Source: CAD feature listing. Evaluate the final solid. Frame: model axes, mm. Face numbers are marked on the shaded views. A direction names the side the tool comes from. Give positions to 0.01 mm unless a question says otherwise; leave off trailing zeros. Loops run counter-clockwise (first coordinate to the right, second up) from the corner with the lowest first, then second, coordinate; pieces in that order, holes last. Notation, with made-up numbers: (-17.75, 29) -> (30.25, 29) arc R16 cw to (30.25, 47) -> close; hole circle Ø8 at (51, 17). An arc over 180 degrees is marked (long way). Return JSON: item names as keys, results as strings. Group by question number.
(1) Cut plane C-C on z = 12.5. Return loops of the section in (x, y).
(2) Cut plane B-B on x = 18. Return loops of the section in (y, z).
(3) Ray query, line 1 (Z direction, x = 26.5, y = 9.5); line 2 (X direction, y = 4.75, z = 27); line 3 (X direction, y = 7.5, z = 51). Return the intervals inside material, ascending. Write a range as from..to.
(4) Cut plane A-A on z = 24.5. Return loops of the section in (x, y), then the cut area to 3 significant figures.
(5) Access query for the marked faces 1, 2, 3, 4 and 5. Directions: +Z, -Z, +X, -X, +Y, -Y. A direction counts if a zero-diameter tool reaches every point of the face in a straight line with its end or side. Return the directions, or none.
(6) Pin query (flat end, axial travel): pin 1 (5 mm diameter, centred on y = 2.5, z = 52.5, fed in from -X); pin 2 (2 mm diameter, centred on x = 33, y = 4, fed in from +Z); pin 3 (1.6 mm diameter, centred on x = 14, z = 55.5, fed in from +Y). Return the tip coordinate at first contact, or that it passes through.
(7) Cut plane D-D on x = -8. Return loops of the section in (y, z).
(8) Draft query along Z for the marked faces 6, 7 and 8. Return one class per face: released by +Z, released by -Z, zero draft, split by the parting line, or undercut.
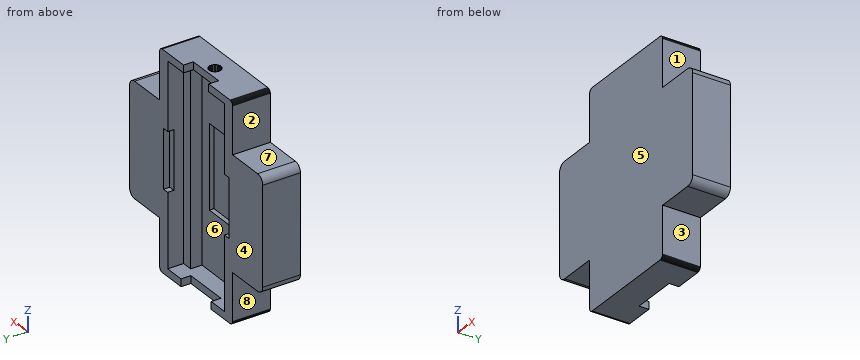
```python
from build123d import *

# Parameters (mm, degrees)
BOSS_EXTRUDE1_DEPTH = 9.999999776
SKETCH2_W           = 17.000000924
SKETCH2_H           = 52.999999374
CUT_EXTRUDE1_DEPTH  = 7.199999876
CUT_EXTRUDE2_REACH  = 66.216
SKETCH4_W           = 2.799998969
SKETCH4_H           = 52.999999374
CUT_EXTRUDE3_REACH  = 66.216
SKETCH6_W           = 2.7999999
SKETCH6_H           = 52.999999374
CUT_EXTRUDE4_REACH  = 66.73
SKETCH7_W           = 10.000000707
SKETCH7_H           = 2.599999774
CUT_EXTRUDE5_REACH  = 66.73
SKETCH8_W           = 12.000000104
SKETCH8_H           = 2.599999774
CUT_EXTRUDE6_DEPTH  = 63.976185295
SKETCH10_W          = 1.699999906
SKETCH10_H          = 15.499999747
CUT_EXTRUDE7_DEPTH  = 1.600000076
SKETCH11_W          = 1.700000837
SKETCH11_H          = 15.499999747
CUT_EXTRUDE8_DEPTH  = 1.600000076
SKETCH12_W          = 11.099998839
SKETCH12_H          = 22.099997848
CUT_EXTRUDE9_DEPTH  = 1.199999941
SKETCH13_W          = 30
SKETCH13_H          = 9.999999776
BOSS_EXTRUDE2_DEPTH = 12
SKETCH14_W          = 30
SKETCH14_H          = 9.999999776
BOSS_EXTRUDE3_DEPTH = 12
FILLET1_R           = 2


with BuildPart() as part:
    # Sketch1 → Boss-Extrude1 (new body)
    with BuildSketch(Plane.XZ):
        Polygon((0.84356498, 0.012312084), (0.999999233, 0), (28.000000864, 0), (28.156435117, 0.012312084), (28.30901742, 0.048942864), (28.453988954, 0.108992681), (28.587784618, 0.190982595), (28.707107529, 0.292893499), (28.80901657, 0.412214547), (28.891006485, 0.546010211), (28.951056302, 0.690983608), (28.987688944, 0.843565969), (28.999999166, 1.000000164), (28.999999166, 56.000001729), (28.987688944, 56.156434119), (28.951056302, 56.309018284), (28.891006485, 56.453991681), (28.80901657, 56.587785482), (28.707107529, 56.707106531), (28.587784618, 56.809015572), (28.453988954, 56.891005486), (28.30901742, 56.951057166), (28.156435117, 56.987687945), (28.000000864, 57.00000003), (0.999999233, 57.00000003), (0.84356498, 56.987687945), (0.690982677, 56.951057166), (0.54600928, 56.891005486), (0.412214547, 56.809015572), (0.292892568, 56.707106531), (0.190982595, 56.587785482), (0.108992681, 56.453991681), (0.048942864, 56.309018284), (0.012311153, 56.156434119), (0, 56.000001729), (0, 1.000000164), (0.012311153, 0.843565969), (0.048942864, 0.690983608), (0.108992681, 0.546010211), (0.190982595, 0.412214547), (0.292892568, 0.292893499), (0.412214547, 0.190982595), (0.54600928, 0.108992681), (0.690982677, 0.048942864), align=None)
    extrude(amount=-BOSS_EXTRUDE1_DEPTH)

    # Sketch2 → Cut-Extrude1 (cut)
    with BuildSketch(Plane(origin=(0, 9.999999776, 0), x_dir=(-1, 0, 0), z_dir=(0, 1, 0))):
        with Locations((-14.499999583, 28.500000015)):
            Rectangle(SKETCH2_W, SKETCH2_H)
    extrude(amount=-CUT_EXTRUDE1_DEPTH, mode=Mode.SUBTRACT)

    # Sketch4 → Cut-Extrude2 (cut, up to next)
    with BuildSketch(Plane.XZ.offset(-5.799999926), mode=Mode.PRIVATE) as cut_extrude2_sk1:
        with Locations((24.39999953, 28.500000015)):
            Rectangle(SKETCH4_W, SKETCH4_H)
    cut_extrude2_tool1 = extrude(cut_extrude2_sk1.sketch, amount=-CUT_EXTRUDE2_REACH, mode=Mode.PRIVATE) & part.part
    add(cut_extrude2_tool1.solids().sort_by_distance((24.4, 5.8, 28.5))[0], mode=Mode.SUBTRACT)

    # Sketch6 → Cut-Extrude3 (cut, up to next)
    with BuildSketch(Plane.XZ.offset(-5.799999926), mode=Mode.PRIVATE) as cut_extrude3_sk1:
        with Locations((4.599999171, 28.500000015)):
            Rectangle(SKETCH6_W, SKETCH6_H)
    cut_extrude3_tool1 = extrude(cut_extrude3_sk1.sketch, amount=-CUT_EXTRUDE3_REACH, mode=Mode.PRIVATE) & part.part
    add(cut_extrude3_tool1.solids().sort_by_distance((4.599999, 5.8, 28.5))[0], mode=Mode.SUBTRACT)

    # Sketch7 → Cut-Extrude4 (cut, up to next)
    with BuildSketch(Plane.XY.offset(57.00000003), mode=Mode.PRIVATE) as cut_extrude4_sk1:
        with Locations((14.500000049, 8.699999889)):
            Rectangle(SKETCH7_W, SKETCH7_H)
    cut_extrude4_tool1 = extrude(cut_extrude4_sk1.sketch, amount=-CUT_EXTRUDE4_REACH, mode=Mode.PRIVATE) & part.part
    add(cut_extrude4_tool1.solids().sort_by_distance((14.5, 8.7, 57))[0], mode=Mode.SUBTRACT)

    # Sketch8 → Cut-Extrude5 (cut, up to next)
    with BuildSketch(Plane(origin=(0, 0, 0), x_dir=(-1, 0, 0), z_dir=(0, 0, -1)), mode=Mode.PRIVATE) as cut_extrude5_sk1:
        with Locations((-14.500000514, 8.699999889)):
            Rectangle(SKETCH8_W, SKETCH8_H)
    cut_extrude5_tool1 = extrude(cut_extrude5_sk1.sketch, amount=-CUT_EXTRUDE5_REACH, mode=Mode.PRIVATE) & part.part
    add(cut_extrude5_tool1.solids().sort_by_distance((14.500001, 8.7, 0))[0], mode=Mode.SUBTRACT)

    # Sketch9 → Cut-Extrude6 (cut, through all)
    with BuildSketch(Plane(origin=(0, 0, 54.999999702), x_dir=(-1, 0, 0), z_dir=(0, 0, -1))):
        Polygon((-16.008604318, 4.466976505), (-15.896821395, 4.219688009), (-15.74485749, 3.994848114), (-15.557079576, 3.798924387), (-15.338891186, 3.637553426), (-15.096570365, 3.515377408), (-14.837087132, 3.435911611), (-14.567905106, 3.401441732), (-14.296771027, 3.412959399), (-14.03148286, 3.470133292), (-13.779673725, 3.571318695), (-13.548586518, 3.713604528), (-13.344869949, 3.892897861), (-13.174383901, 4.104040563), (-13.042034581, 4.34095785), (-12.951626442, 4.596835002), (-12.905763462, 4.86431038), (-12.905763462, 5.135689396), (-12.951626442, 5.403164774), (-13.042034581, 5.659041926), (-13.174383901, 5.895959679), (-13.344869949, 6.107102148), (-13.548586518, 6.286395248), (-13.779673725, 6.428681314), (-14.03148286, 6.529866718), (-14.296771027, 6.587040611), (-14.567905106, 6.598558277), (-14.837087132, 6.564088166), (-15.096570365, 6.484622601), (-15.338891186, 6.362446584), (-15.557079576, 6.201075856), (-15.74485749, 6.005152129), (-15.896821395, 5.780311767), (-16.008604318, 5.533023737), (-16.076983884, 5.270401482), (-16.10000059, 4.999999888), (-16.076983884, 4.729599226), align=None)
    extrude(amount=-CUT_EXTRUDE6_DEPTH, mode=Mode.SUBTRACT)

    # Sketch10 → Cut-Extrude7 (cut)
    with BuildSketch(Plane(origin=(0, 9.999999776, 0), x_dir=(-1, 0, 0), z_dir=(0, 1, 0))):
        with Locations((-2.349999268, 29.250000603)):
            Rectangle(SKETCH10_W, SKETCH10_H)
    extrude(amount=-CUT_EXTRUDE7_DEPTH, mode=Mode.SUBTRACT)

    # Sketch11 → Cut-Extrude8 (cut)
    with BuildSketch(Plane(origin=(0, 9.999999776, 0), x_dir=(-1, 0, 0), z_dir=(0, 1, 0))):
        with Locations((-26.649999433, 29.250000603)):
            Rectangle(SKETCH11_W, SKETCH11_H)
    extrude(amount=-CUT_EXTRUDE8_DEPTH, mode=Mode.SUBTRACT)

    # Sketch12 → Cut-Extrude9 (cut)
    with BuildSketch(Plane(origin=(0, 2.7999999, 0), x_dir=(-1, 0, 0), z_dir=(0, 1, 0))):
        with Locations((-14.499999117, 28.500000015)):
            Rectangle(SKETCH12_W, SKETCH12_H)
    extrude(amount=-CUT_EXTRUDE9_DEPTH, mode=Mode.SUBTRACT)

    # Sketch13 → Boss-Extrude2 (add)
    with BuildSketch(Plane.ZY):
        with Locations((28.500000946, 4.999999888)):
            Rectangle(SKETCH13_W, SKETCH13_H)
    extrude(amount=BOSS_EXTRUDE2_DEPTH)

    # Sketch14 → Boss-Extrude3 (add)
    with BuildSketch(Plane(origin=(28.999999166, 0, 0), x_dir=(0, 0, -1), z_dir=(1, 0, 0))):
        with Locations((-28.500000946, 4.999999888)):
            Rectangle(SKETCH14_W, SKETCH14_H)
    extrude(amount=BOSS_EXTRUDE3_DEPTH)

    # Fillet1
    fillet1_edges = [part.edges().sort_by_distance(p)[0] for p in [
        (-12, 4.999999888, 13.500000946),
        (-12, 4.999999888, 43.500000946),
        (40.999999166, 4.999999888, 43.500000946),
        (40.999999166, 4.999999888, 13.500000946),
    ]]
    fillet(fillet1_edges, radius=FILLET1_R)


solid = part.part
```
Answers:
{
 "1": {"outline": "(0, 0) -> (29, 0) -> (29, 10) -> (25.8, 10) -> (25.8, 5.8) -> (23, 5.8) -> (23, 2.8) -> (6, 2.8) -> (6, 5.8) -> (3.2, 5.8) -> (3.2, 10) -> (0, 10) -> close"},
 "2": {"outline": "(0, 0) -> (7.4, 0) -> (7.4, 2) -> (2.8, 2) -> (2.8, 17.45) -> (1.6, 17.45) -> (1.6, 39.55) -> (2.8, 39.55) -> (2.8, 55) -> (7.4, 55) -> (7.4, 57) -> (0, 57) -> close"},
 "3": {"line 1": "0..21.5, 37..57", "line 2": "-12..6, 23..41", "line 3": "0..3.2, 25.8..29"},
 "4": {"outline": "(-12, 0) -> (41, 0) -> (41, 10) -> (27.5, 10) -> (27.5, 8.4) -> (25.8, 8.4) -> (25.8, 5.8) -> (23, 5.8) -> (23, 2.8) -> (20.05, 2.8) -> (20.05, 1.6) -> (8.95, 1.6) -> (8.95, 2.8) -> (6, 2.8) -> (6, 5.8) -> (3.2, 5.8) -> (3.2, 8.4) -> (1.5, 8.4) -> (1.5, 10) -> (-12, 10) -> close", "area": "365 mm²"},
 "5": {"face 1": "+Z, +X, +Y, -Y", "face 2": "+Z, -X, +Y, -Y", "face 3": "-Z, +X, +Y, -Y", "face 4": "+Z, -Z, +X, -X, +Y", "face 5": "+Z, -Z, +X, -X, -Y"},
 "6": {"pin 1": "x = 0", "pin 2": "z = 43.5", "pin 3": "y = 7.4"},
 "7": {"outline": "(0, 13.5) -> (10, 13.5) -> (10, 43.5) -> (0, 43.5) -> close"},
 "8": {"face 6": "undercut", "face 7": "released by +Z", "face 8": "zero draft"}
}
